```python
from build123d import *

# Parameters (mm, degrees)
CHANFREIN1_SIZE         = 0.5
ENL_V_MAT_EXTRU_2_DEPTH = 3


with BuildPart() as part:
    # Esquisse1 → Révolution1 (revolve)
    with BuildSketch(Plane.XY, mode=Mode.PRIVATE) as r_volution1_sk:
        Polygon((1.5, 7.9), (5.925, 7.9), (5.925, 6.9), (3.925, 6.9), (3.925, 0), (1.5, 0), align=None)
    revolve(r_volution1_sk.sketch.rotate(Axis((0, 0, 0), (0, 1, 0)), 90), axis=Axis((0, 0, 0), (0, 1, 0)))

    # Chanfrein1
    chanfrein1_edges = [part.edges().sort_by_distance(p)[0] for p in [
        (0, 0, 3.925),
        (0, 6.9, 3.925),
    ]]
    chamfer(chanfrein1_edges, length=CHANFREIN1_SIZE)

    # Esquisse3 → Enlèv. mat.-Extru.2 (cut)
    with BuildSketch(Plane(origin=(0, 7.9, 0), x_dir=(1, 0, 0), z_dir=(0, 1, 0))):
        Polygon((1.58771324, 2.75), (-1.58771324, 2.75), (-3.175426481, 0), (-1.58771324, -2.75), (1.58771324, -2.75), (3.175426481, 0), align=None)
    extrude(amount=-ENL_V_MAT_EXTRU_2_DEPTH, mode=Mode.SUBTRACT)


solid = part.part
```
The model under review builds one solid part; all positions refer to its coordinate system, in mm. A direction names the side the tool comes from. Give positions to 0.01 mm unless a question says otherwise; leave off trailing zeros. Write each loop counter-clockwise with the first axis right and the second up, starting at its lowest first coordinate (ties: lowest second). Pieces come first, ordered by that corner, then holes. Notation, with made-up numbers: (29, -25.5) -> (83, -25.5) arc R27 ccw to (83, -7.5) -> close; hole circle Ø2 at (40, 61). An arc over 180 degrees is marked (long way). Answer in a Markdown table with one row per item.
1) Add section D-D on z = -5. State the section outline as (x, y) points.
Worked answers:
| item | result |
|---|---|
| outline | (-3.18, 6.9) -> (3.18, 6.9) -> (3.18, 7.9) -> (-3.18, 7.9) -> close |
2) Mouldability with a two-part tool opening along Z and no side actions: class faces 1 (the cylindrical face through (3.83, 3.41, 0.85)), 2 (the flat face through (3, 7.9, 1)), 3 (the cylindrical face through (-0.45, 2.48, -1.43)) as +Z half, -Z half, draft (parallel to the pull), parting line (faces both ways), or undercut.
Worked answers:
| item | result |
|---|---|
| face 1 | parting line |
| face 2 | draft |
| face 3 | undercut |
3) Clearance check with flat-ended pins moving along their axes: P1, Ø2, axis at y = 1, z = -2.5, coming from the +X side; P2, Ø2, axis at y = 5, z = 2, coming from the +X side; P3, Ø1.5, axis at x = -1, y = 6, coming from the -Z side. State where each tip first meets the part, or that it passes through.
Worked answers:
| item | result |
|---|---|
| P1 | x = 3.63 |
| P2 | x = 3.8 |
| P3 | z = -4.17 |
4) Tool access review of faces 4 (the flat face through (0.7, 0, -1.5)), 5 (the flat face through (-2.37, 6.421, -1.394)): name each direction out of +Z, -Z, +X, -X, +Y, -Y from which nothing blocks a thin tool from reaching the whole face with its end or side.
Worked answers:
| item | result |
|---|---|
| face 4 | +Z, -Z, +X, -X, -Y |
| face 5 | +Y |
5) Add section B-B on y = 5.5. State the section outline as (x, z) points (3 decimals), plus the area to 3 significant figures.
Worked answers:
| item | result |
|---|---|
| outline | circle Ø7.85 at (0, 0); hole (-3.175, 0) -> (-1.588, -2.75) -> (1.588, -2.75) -> (3.175, 0) -> (1.588, 2.75) -> (-1.588, 2.75) -> close |
| area | 22.2 mm² |
6) For L1, parallel to X at y = 2.8, z = 0 (3 decimals); L2, parallel to Y at x = -0.5, z = -1.75; L3, parallel to Y at x = -4, z = -3.25, list the stretches that pass through material, from the lowest coordinate up. Write a range as [from, to].
Worked answers:
| item | result |
|---|---|
| L1 | [-3.925, -1.5], [1.5, 3.925] |
| L2 | [0, 4.9] |
| L3 | [6.9, 7.9] |
7) Add section C-C on y = 4. State the section outline as (x, z) points (3 decimals), plus the area to 3 significant figures.
Worked answers:
| item | result |
|---|---|
| outline | circle Ø7.85 at (0, 0); hole circle Ø3 at (0, 0) |
| area | 41.3 mm² |
8) Add section A-A on x = 0. State the section outline as (y, z) points (3 decimals).
Worked answers:
| item | result |
|---|---|
| outline | (0, -3.425) -> (0.5, -3.925) -> (6.4, -3.925) -> (6.9, -4.425) -> (6.9, -5.925) -> (7.9, -5.925) -> (7.9, -2.75) -> (4.9, -2.75) -> (4.9, -1.5) -> (0, -1.5) -> close; (0, 1.5) -> (4.9, 1.5) -> (4.9, 2.75) -> (7.9, 2.75) -> (7.9, 5.925) -> (6.9, 5.925) -> (6.9, 4.425) -> (6.4, 3.925) -> (0.5, 3.925) -> (0, 3.425) -> close |
